Check sheet for the drawn part. Datum: minimum x, y, z corner. Units: mm. Give positions to 0.01 mm unless a question says otherwise; leave off trailing zeros. Order: outer loops, then holes, each group sorted by start corner. A loop starts at its lowest first (then second) coordinate and runs counter-clockwise, first axis right, second up.
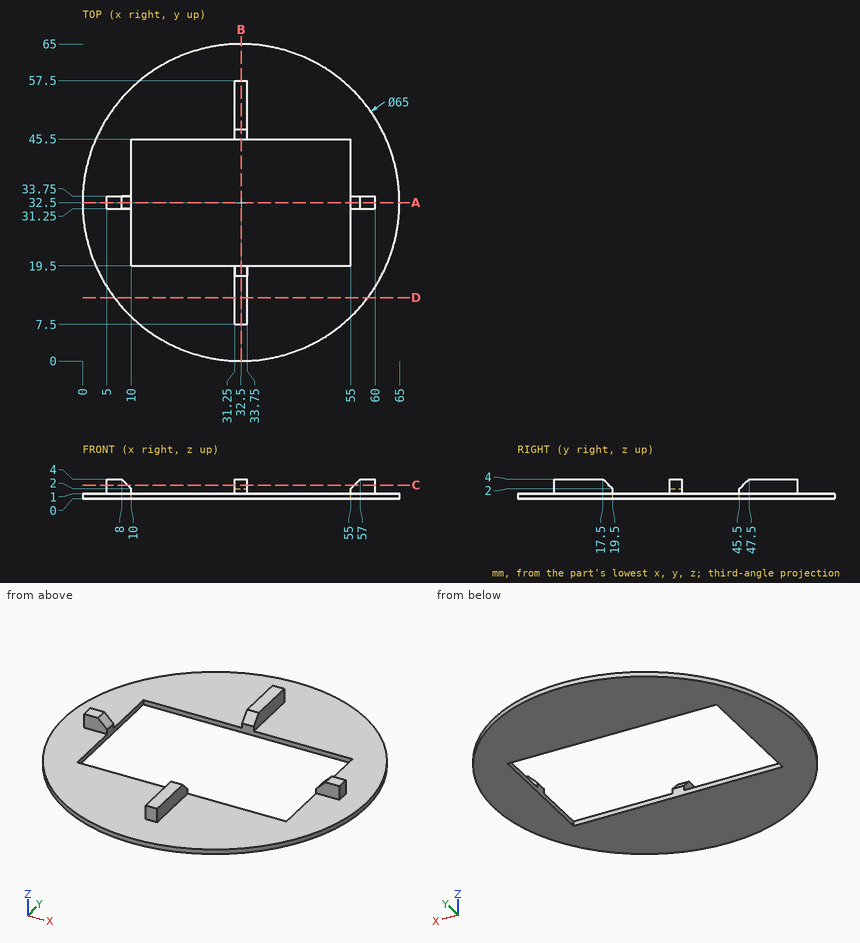
(1) Section check C-C, the plane z = 2.75. Enter the section's corners in (x, y).
Solved:
outline: (5, 31.25) - (9.25, 31.25) - (9.25, 33.75) - (5, 33.75) - close; (31.25, 7.5) - (33.75, 7.5) - (33.75, 18.75) - (31.25, 18.75) - close; (31.25, 46.25) - (33.75, 46.25) - (33.75, 57.5) - (31.25, 57.5) - close; (55.75, 31.25) - (60, 31.25) - (60, 33.75) - (55.75, 33.75) - close
(2) Section check A-A, the plane y = 32.5. Enter the section's corners in (x, z), then the cut area to 3 significant figures.
Solved:
outline: (0, 0) - (10, 0) - (10, 2) - (8, 4) - (5, 4) - (5, 1) - (0, 1) - close; (55, 0) - (65, 0) - (65, 1) - (60, 1) - (60, 4) - (57, 4) - (55, 2) - close
area: 46.0 mm2
(3) Go/stop test with flat-tipped pins: pin 1 (1.5 mm diameter, centred on y = 20.5, z = 3, fed in from -X); pin 2 (2 mm diameter, centred on x = 54, y = 7, fed in from +Z); pin 3 (2 mm diameter, centred on x = 33, z = 2.5, fed in from +Y); pin 4 (0.8 mm diameter, centred on y = 33, z = 3, fed in from +X). Record where each tip stops, or that it passes through.
Solved:
pin 1: passes through
pin 2: stops at z = 1
pin 3: stops at y = 57.5
pin 4: stops at x = 60
(4) Section check D-D, the plane y = 13. Enter the section's corners in (x, z), then the cut area to 3 significant figures.
Solved:
outline: (6.5, 0) - (58.5, 0) - (58.5, 1) - (33.75, 1) - (33.75, 4) - (31.25, 4) - (31.25, 1) - (6.5, 1) - close
area: 59.5 mm2
(5) Scan lines: line 1 (X direction, y = 33.5, z = 1.7); line 2 (Z direction, x = 48.5, y = 56.5); line 3 (Y direction, x = 17, z = 0.55). Record each from-to range of solid material in increasing order.
Solved:
line 1: x = 5 to 10, 55 to 60
line 2: z = 0 to 1
line 3: y = 3.93 to 19.5, 45.5 to 61.07
(6) Section check B-B, the plane x = 32.5. Enter the section's corners in (y, z), then the cut area to 3 significant figures.
Solved:
outline: (0, 0) - (19.5, 0) - (19.5, 2) - (17.5, 4) - (7.5, 4) - (7.5, 1) - (0, 1) - close; (45.5, 0) - (65, 0) - (65, 1) - (57.5, 1) - (57.5, 4) - (47.5, 4) - (45.5, 2) - close
area: 107 mm2
